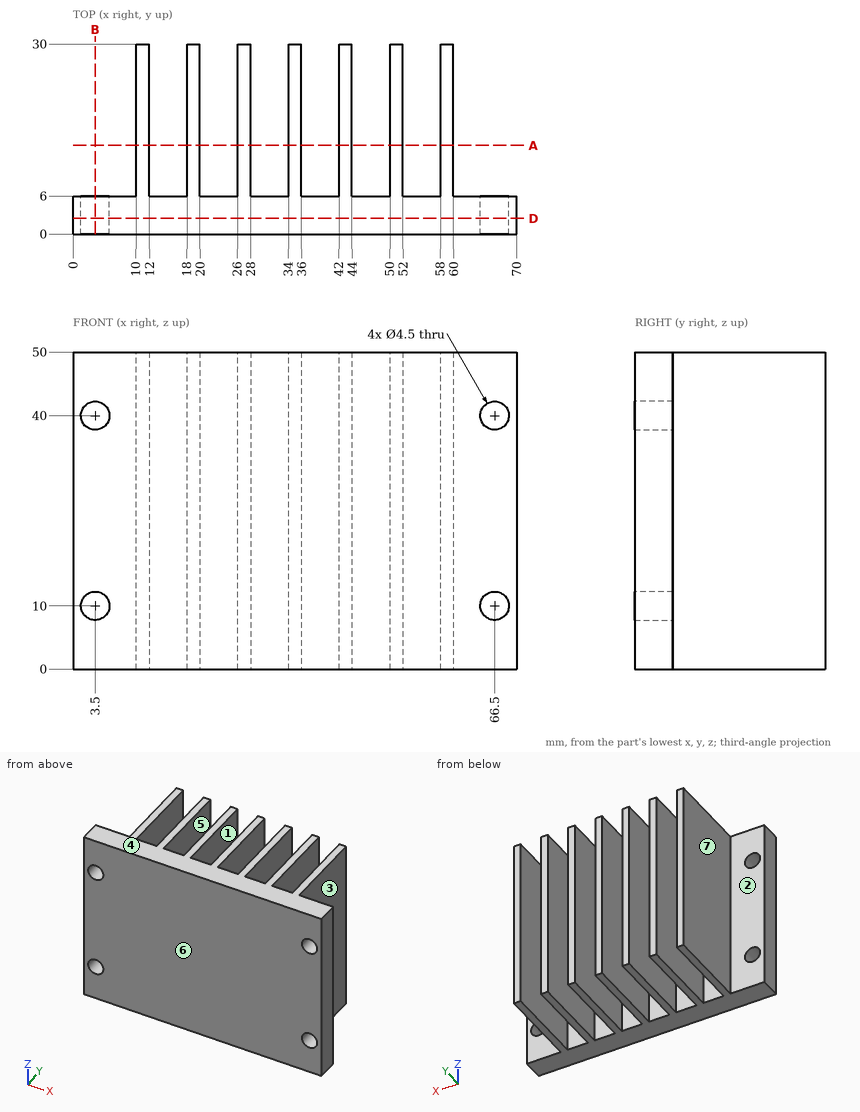
Study the drawing (mm; zero at the part's minimum x, y, z) and answer. A direction names the side the tool comes from. Round coordinates to 2 decimals unless told otherwise and drop trailing zeros. Order: outer loops, then holes, each group sorted by start corner. A loop starts at its lowest first (then second) coordinate and runs counter-clockwise, first axis right, second up. Notation, with made-up numbers: (57.25, 73) -> (75.25, 73) arc R30 ccw to (75.25, 100) -> close; hole circle Ø11 at (28.25, -17.5). An arc over 180 degrees is marked (long way). Write each question's results on one line, items separated by ' | '. Start each with the question number.
Q1. Each of these flat-tipped pins is pushed along its axis until it touches: pin 1 (1 mm diameter, centred on y = 14.5, z = 39, fed in from -X); pin 2 (1.8 mm diameter, centred on x = 15, z = 32.5, fed in from +Y); pin 3 (12 mm diameter, centred on y = 23, z = 23.5, fed in from +X). Where does it stop, or does it pass through?
Q2. Find section A-A (y = 14). Determine the outline of the cut face in (x, z), then the cut area to 3 significant figures.
Q3. Which of the six approach directions +Z, -Z, +X, -X, +Y, -Y give full straight-line access (tool end or side, diameter ignored) to the marked faces 1, 2, 3 and 4?
Q4. Find section B-B (x = 3.5). Determine the outline of the cut face in (y, z), then the cut area to 3 significant figures.
Q5. Find section D-D (y = 2.5). Determine the outline of the cut face in (x, z), then the cut area to 3 significant figures.
Q6. Straight lines are drawn through the part: probe 1 along X at (y, z) = (4.7, 10); probe 2 along Y at (x, z) = (53.5, 5). For each, find the intervals that lie inside material, in ascending order. Write a range as from..to.
Q7. The mould has two halves that part along X. Classify the marked faces 5, 6 and 7: pulls with the +X half, pulls with the -X half, needs draft (parallel to the pull), parting line crosses it, or undercut.
Worked answers:
1) pin 1: stops at x = 10 | pin 2: stops at y = 6 | pin 3: stops at x = 60
2) outline: (10, 0) -> (12, 0) -> (12, 50) -> (10, 50) -> close; (18, 0) -> (20, 0) -> (20, 50) -> (18, 50) -> close; (26, 0) -> (28, 0) -> (28, 50) -> (26, 50) -> close; (34, 0) -> (36, 0) -> (36, 50) -> (34, 50) -> close; (42, 0) -> (44, 0) -> (44, 50) -> (42, 50) -> close; (50, 0) -> (52, 0) -> (52, 50) -> (50, 50) -> close; (58, 0) -> (60, 0) -> (60, 50) -> (58, 50) -> close | area: 700 mm2
3) face 1: +Z, -Z, +Y | face 2: +Z, -Z, -X, +Y | face 3: +Z, -Z, +X, +Y | face 4: +Z, +X, -X, +Y, -Y
4) outline: (0, 0) -> (6, 0) -> (6, 7.75) -> (0, 7.75) -> close; (0, 12.25) -> (6, 12.25) -> (6, 37.75) -> (0, 37.75) -> close; (0, 42.25) -> (6, 42.25) -> (6, 50) -> (0, 50) -> close | area: 246 mm2
5) outline: (0, 0) -> (70, 0) -> (70, 50) -> (0, 50) -> close; hole circle Ø4.5 at (3.5, 10); hole circle Ø4.5 at (3.5, 40); hole circle Ø4.5 at (66.5, 10); hole circle Ø4.5 at (66.5, 40) | area: 3,440 mm2
6) probe 1: x = 0..1.25, 5.75..64.25, 68.75..70 | probe 2: y = 0..6
7) face 5: undercut | face 6: needs draft | face 7: pulls with the -X half
